Can you work these out from the model? Positions are in its coordinate system, mm. Face numbers are marked on the shaded views. A direction names the side the tool comes from. Coordinates: 2 decimals unless noted, no trailing zeros. Order: outer loops, then holes, each group sorted by start corner. A loop starts at its lowest first (then second) coordinate and runs counter-clockwise, first axis right, second up. Notation, with made-up numbers: (32.5, -18) -> (85.5, -18) arc R22 ccw to (85.5, -3) -> close; hole circle Ø6 at (7, 78.25). An arc over 180 degrees is marked (long way). Use a Markdown table: item, result. Add a question column.
1. For the marked faces 4, 5 and 6, which set-ups out of +Z, -Z, +X, -X, +Y, -Y let a thin tool reach every point of the face, with its end or its side?
2. We'd pull the mould along Y, two halves only. Please class the marked faces 1, 2 and 3: pulls with the +Y half, pulls with the -Y half, needs draft (parallel to the pull), parting line crosses it, or undercut.
3. Suppose I cut it at A-A, the plane z = 12. List the corners of the cut face in (x, y) for me, then the cut area to 3 significant figures.
4. For pin 1 Ø1.3 at (y, z) = (0.5, 11.5) entering from -X; pin 2 Ø1 at (x, y) = (1.5, -2.5) entering from -Z; pin 3 Ø1 at (x, z) = (-3, 11) entering from +Y; pin 4 Ø1.5 at (y, z) = (2.5, 2) entering from -X, each with a flat end and sliding along its axis, tell me the tip position at first contact or that it passes through.
5. If I drill on line 1 along Y through (x, z) = (0, 15.2); line 2 along Z through (x, y) = (0, 5); line 3 along Y through (x, z) = (-0.5, 8.25) (3 decimals), over which ranges is the centre line in solid material (lowest first)? Write a range as from..to.
Autodesk Inventor part; units mm, degrees
ref_plane "YZ Plane" through (0, 0, 0) normal (1, 0, 0) x (0, 1, 0)
ref_plane "XZ Plane" through (0, 0, 0) normal (0, 1, 0) x (-1, 0, 0)
ref_plane "XY Plane" through (0, 0, 0) normal (0, 0, 1) x (1, 0, 0)
sketch "Sketch1" plane through (0, 0, 0) normal (0, 0, 1) x (1, 0, 0)
  circle A0 centre (0, 0) radius 3
  dimension "d0" = 6
extrude "Extrusion1" add sketch "Sketch1" along normal blind 5
sketch "Sketch2" plane through (0, 0, 5) normal (0, 0, 1) x (1, 0, 0)
  circle A0 centre (0, 0) radius 3.775
  dimension "d3" = 7.55
extrude "Extrusion2" add sketch "Sketch2" along normal blind 3
sketch "Sketch3" plane through (0, 0, 8) normal (0, 0, 1) x (1, 0, 0)
  circle A0 centre (0, 0) radius 7
  circle A1 centre (0, 0) radius 2.8
  dimension "d7" = 14
  dimension "d25" = 5.6
extrude "Extrusion3" add sketch "Sketch3" along normal blind 2.2
sketch "Sketch5" plane through (0, 0, 10.2) normal (0, 0, 1) x (1, 0, 0)
  line L0 (-4.15, 2.396) -> (0, 4.792)
  line L1 (0, 4.792) -> (4.15, 2.396)
  line L2 (4.15, 2.396) -> (4.15, -2.396)
  line L3 (4.15, -2.396) -> (0, -4.792)
  line L4 (0, -4.792) -> (-4.15, -2.396)
  line L5 (-4.15, -2.396) -> (-4.15, 2.396)
  circle A0 centre (0, 0) radius 7
  dimension "d19" = 8.3
extrude "Extrusion5" add sketch "Sketch5" along normal blind 4.3
sketch "Sketch6" plane through (0, 0, 14.5) normal (0, 0, 1) x (1, 0, 0)
  circle A0 centre (0, 0) radius 7
  circle A1 centre (0, 0) radius 2.8
  dimension "d24" = 5.6
extrude "Extrusion6" add sketch "Sketch6" along normal blind 0.9
chamfer "Chamfer1" distance 1 angle 45 1 edges at (-3, 0, 0)
chamfer "Chamfer2" distance 0.7 angle 45 2 edges at (-3.775, 0, 5) (-7, 0, 8)
equation "\"m3_hex_s\" = 5.4"
equation "\"m3_hex_m\" = 2.3"
equation "\"m3_rund_d\" = 5.95"
equation "\"m3_rund_m\" = 2.6"
equation "\"l______________l\" = 0"
equation "\"Lengths\" = 0"
equation "\"L20\" = 0"
equation "\"L25\" = 0"
equation "\"L16\" = 0"
equation "\"L12\" = 0"
equation "\"L8\" = 0"
equation "\"L4\" = 0"
equation "\"m3_s\" = 5.4"
equation "\"m3_m\" = 2.3"
properties part number "Shaft_to_beam_interface_3DPrint"
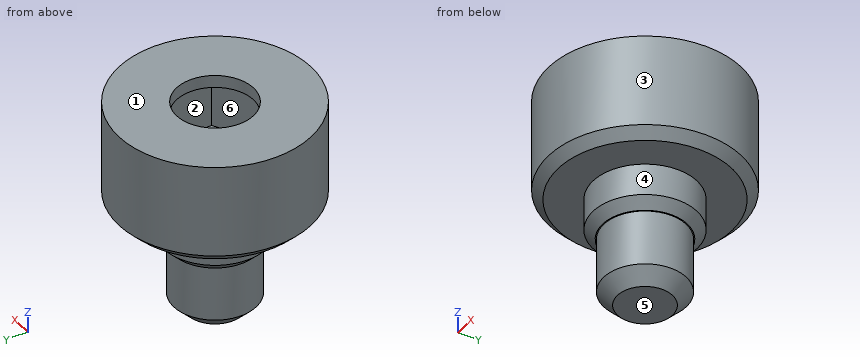
Worked out:
| question | item | result |
|---|---|---|
| 1 | face 4 | -Z |
| 1 | face 5 | -Z, +X, -X, +Y, -Y |
| 1 | face 6 | none |
| 2 | face 1 | needs draft |
| 2 | face 2 | undercut |
| 2 | face 3 | parting line crosses it |
| 3 | outline | circle Ø14 at (0, 0); hole (-4.15, -2.4) -> (0, -4.79) -> (4.15, -2.4) -> (4.15, 2.4) -> (0, 4.79) -> (-4.15, 2.4) -> close |
| 3 | area | 94.3 mm² |
| 4 | pin 1 | stops at x = -7 |
| 4 | pin 2 | stops at z = 0.42 |
| 4 | pin 3 | stops at y = 6.54 |
| 4 | pin 4 | stops at x = -2.44 |
| 5 | line 1 | y = -7..-2.8, 2.8..7 |
| 5 | line 2 | z = 8..15.4 |
| 5 | line 3 | y = -6.531..-2.755, 2.755..6.531 |
